Can you work these out from the drawing? Everything is in mm from the part's minimum corner. Coordinates: 2 decimals unless noted, no trailing zeros. Write each loop counter-clockwise with the first axis right and the second up, starting at its lowest first coordinate (ties: lowest second). Pieces come first, ordered by that corner, then holes. Notation, with made-up numbers: (76.5, -26) -> (120.5, -26) arc R32 ccw to (120.5, 10) -> close; hole circle Ø1 at (-7, 25). An arc over 180 degrees is marked (long way). Answer as CSV lines item,"result". Start each with the question number.
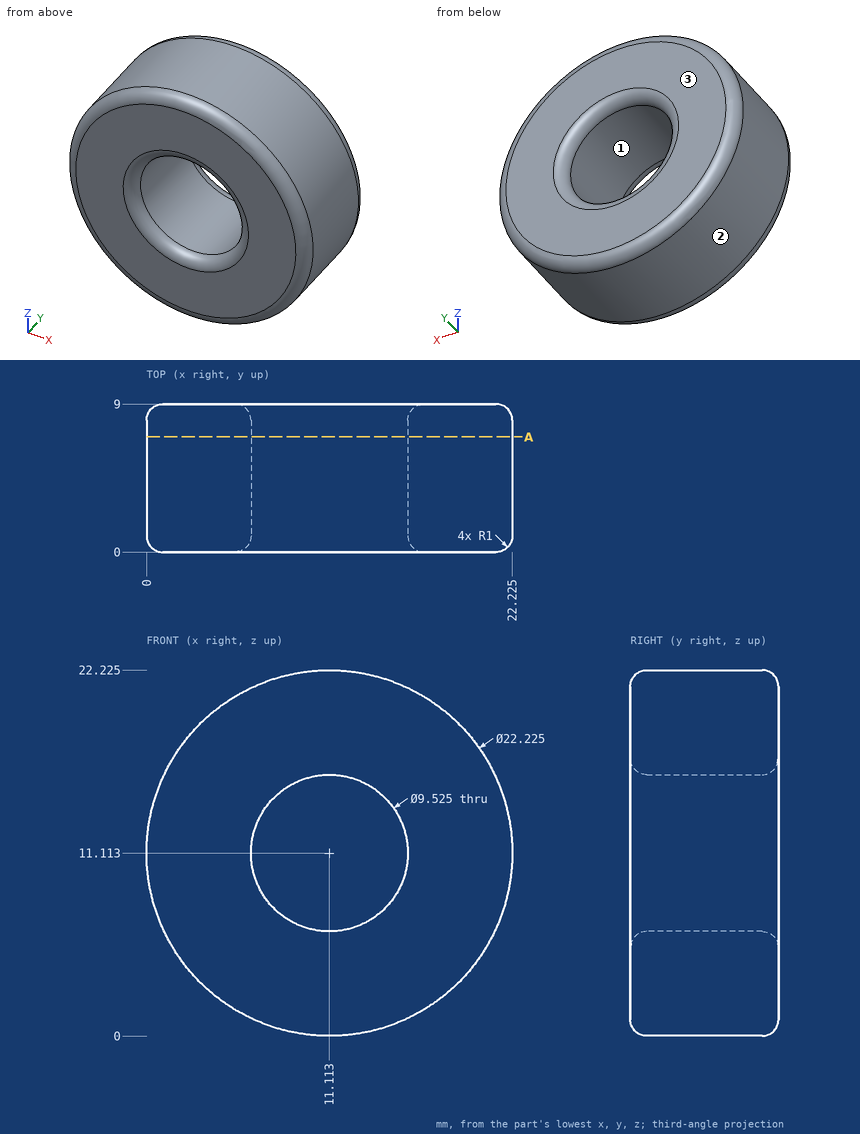
Q1. If we mould it in two halves opening along Z, with no side actions, what happens to the marked faces 1, 2 and 3? For each: released by +Z, released by -Z, zero draft, split by the parting line, or undercut.
Q2. For pin 1 (1 mm diameter, centred on x = 17.5, z = 2.5, fed in from +Y); pin 2 (2 mm diameter, centred on x = 12.5, y = 8, fed in from +Z); pin 3 (1 mm diameter, centred on x = 7, y = 5.5, fed in from -Z); pin 4 (7.5 mm diameter, centred on x = 11.11, z = 11.11, fed in from +Y), each with a flat end and sliding along its axis, tell me the tip position at first contact or that it passes through.
Q3. Imagine slicing it at A-A (y = 7). Write out the boundary of the cut face in (x, z) (1 decimal).
Q4. I need wall thicknesses on L1, parallel to Z at x = 11, y = 6 (1 decimal); L2, parallel to X at y = 0.75, z = 7.5 (1 decimal); L3, parallel to Y at x = 3, z = 17.25. Which ranges of each line are inside material? Lowest first, please.
Entries:
1,face 1,"undercut"
1,face 2,"split by the parting line"
1,face 3,"zero draft"
2,pin 1,"y = 8.99"
2,pin 2,"z = 22.22"
2,pin 3,"z = 0.6"
2,pin 4,"through"
3,outline,"circle Ø22.2 at (11.1, 11.1); hole circle Ø9.5 at (11.1, 11.1)"
4,L1,"0 to 6.4, 15.9 to 22.2"
4,L2,"0.6 to 8, 14.3 to 21.6"
4,L3,"0 to 9"
